For this review, use the dimensioned drawing (mm, ordinates from the lowest corner) and the shaded views. A direction names the side the tool comes from. Coordinates: 2 decimals unless noted, no trailing zeros. Loops run counter-clockwise (first coordinate to the right, second up) from the corner with the lowest first, then second, coordinate; pieces in that order, holes last.
1. Take a section at C-C, the plane x = 1.25. State the section outline as (y, z) points.
2. Take a section at B-B, the plane z = 6. State the section outline as (x, y) points.
3. Clearance check with flat-ended pins moving along their axes: P1, Ø2.5, axis at y = 2, z = 2, coming from the -X side; P2, Ø1.6, axis at x = 4, y = 4, coming from the -Z side; P3, Ø0.6, axis at x = 7, z = 5, coming from the -Y side; P4, Ø2, axis at x = 6.5, z = 1, coming from the -Y side. State where each tip first meets the part, or that it passes through.
4. Take a section at A-A, the plane y = 2. State the section outline as (x, z) points, then the cut area to 3 significant figures.
5. To check wall thickness, follow probe 1 along Y at (x, z) = (1.2, 6); probe 2 along X at (y, z) = (6.5, 3.5); probe 3 along Z at (x, y) = (5, 1). State the ranges of each line that lie inside material, in increasing order.
6. Machinability: for the marked faces 1, 2, 3 and 4, which of the approach directions +Z, -Z, +X, -X, +Y, -Y give a long, thin tool a straight path to every point of the face, cutting with its end or side? Answer none if there is none.
7. Take a section at D-D, the plane y = 9.25. State the section outline as (x, z) points.
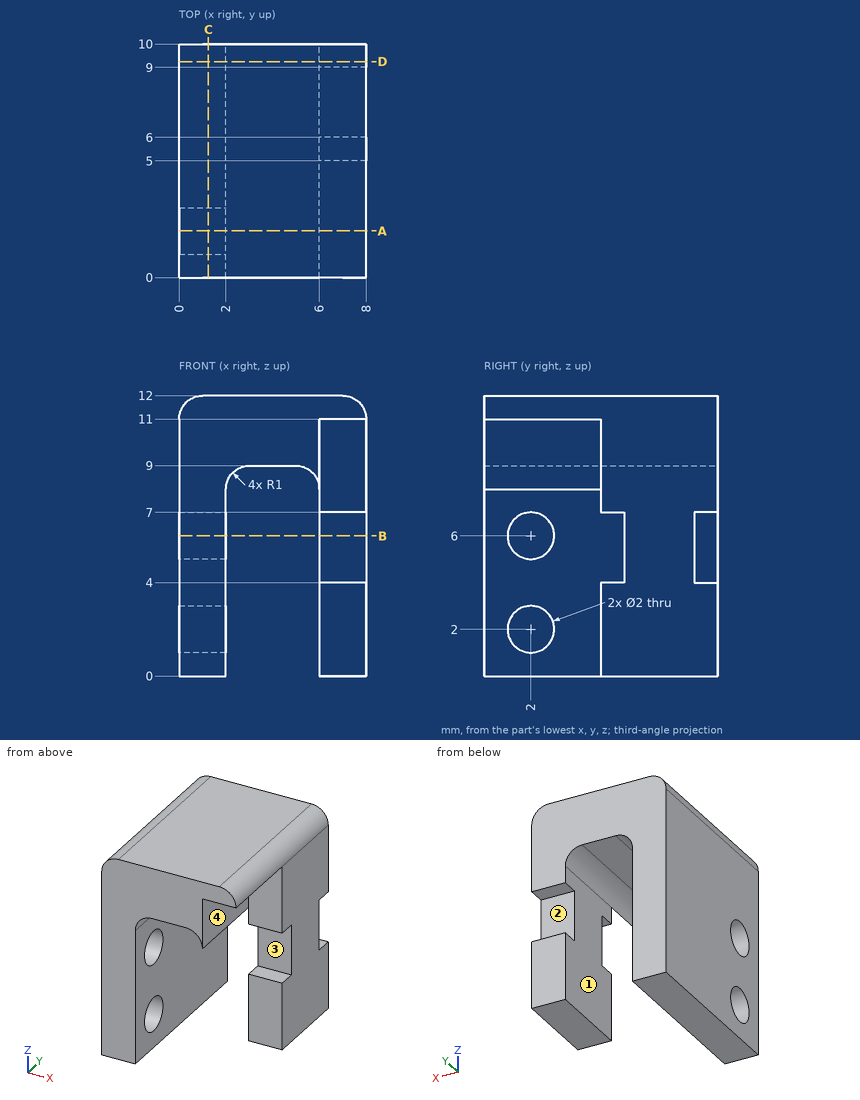
Results list:
1. outline: (0, 0) - (10, 0) - (10, 12) - (0, 12) - close; hole circle Ø2 at (2, 2); hole circle Ø2 at (2, 6)
2. outline: (0, 0) - (2, 0) - (2, 1) - (0, 1) - close; (0, 3) - (2, 3) - (2, 10) - (0, 10) - close; (6, 6) - (8, 6) - (8, 9) - (6, 9) - close
3. P1: stops at x = 0
3. P2: stops at z = 9
3. P3: stops at y = 6
3. P4: stops at y = 5
4. outline: (0, 0) - (2, 0) - (2, 1) - (0, 1) - close; (0, 3) - (2, 3) - (2, 5) - (0, 5) - close; (0, 7) - (2, 7) - (2, 8) arc R1 cw to (3, 9) - (5, 9) arc R1 cw to (6, 8) - (6, 11) - (8, 11) arc R1 ccw to (7, 12) - (1, 12) arc R1 ccw to (0, 11) - close
4. area: 30.0 mm2
5. probe 1: y = 0 to 1, 3 to 10
5. probe 2: x = 0 to 2, 6 to 8
5. probe 3: z = 9 to 12
6. face 1: -Z, +Y, -Y
6. face 2: +X, +Y
6. face 3: +X, -Y
6. face 4: -Z, +X, -Y
7. outline: (0, 0) - (2, 0) - (2, 8) arc R1 cw to (3, 9) - (5, 9) arc R1 cw to (6, 8) - (6, 7) - (8, 7) - (8, 11) arc R1 ccw to (7, 12) - (1, 12) arc R1 ccw to (0, 11) - close; (6, 0) - (8, 0) - (8, 4) - (6, 4) - close
